```python
from build123d import *

# Parameters (mm, degrees)
F0_W     = 838.2
F0_H     = 457.2
F0_W_2   = 685.8
F0_H_2   = 304.8
F1_DEPTH = 22.225
F2_DEPTH = 9.525
F4_DEPTH = 6.35
F6_DEPTH = 6.35


with BuildPart() as f1:
    # F0 (on Front) → F1 (new body, symmetric)
    with BuildSketch(Plane.XZ):
        Rectangle(F0_W, F0_H)
        Rectangle(F0_W_2, F0_H_2, mode=Mode.SUBTRACT)
    extrude(amount=F1_DEPTH, both=True)

    # F0 (on Front) → F2 (join, symmetric)
    with BuildSketch(Plane.XZ):
        Rectangle(F0_W_2, F0_H_2)
    extrude(amount=F2_DEPTH, both=True)

    # F3 (on face) → F4 (join)
    with BuildSketch(Plane.XZ.offset(9.525)):
        Polygon((342.9, -152.4), (-189.5254737066, 152.4), (-342.9, 152.4), (189.5254737066, -152.4), align=None)
    extrude(amount=F4_DEPTH)

    # F5 (on face) → F6 (join)
    with BuildSketch(Plane.XZ.offset(9.525)):
        Polygon((-76.6872631467, 0), (-342.9, -152.4), (-189.5254737066, -152.4), (0, -43.90150164), align=None)
        Polygon((342.9, 152.4), (189.5254737066, 152.4), (0, 43.90150164), (76.6872631467, 0), align=None)
    extrude(amount=F6_DEPTH)


solid = f1.part
```
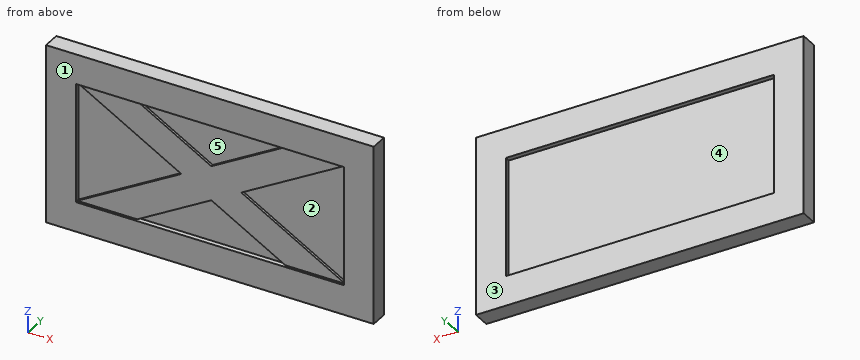
Could you check a few things on this model? Use its own coordinates, in mm. Face numbers are marked on the shaded views. A direction names the side the tool comes from. Round coordinates to 2 decimals unless told otherwise and drop trailing zeros. Loops run counter-clockwise (first coordinate to the right, second up) from the corner with the lowest first, then second, coordinate; pieces in that order, holes last. Notation, with made-up numbers: (62.5, 65) - (95.5, 65) arc R13 ccw to (95.5, 88) - close; hole circle Ø1 at (55, -35). An arc over 180 degrees is marked (long way). Answer in a Markdown table with one row per item. Add a question column.
(1) I need wall thicknesses on line 1 along Z through (x, y) = (-109, -20); line 2 along X through (y, z) = (20, -11.5); line 3 along X through (y, z) = (-10.5, 58.5). Which ranges of each line are inside material? Lowest first, please.
(2) If we section it at A-A (x = 40): Please give me the cut outline in (y, z) (3 decimals), plus the area to 3 significant figures.
(3) I'm going to push flat-ended pins straight in: pin 1 (6 mm diameter, centred on x = -141.5, z = 90, fed in from +Y) (3 decimals); pin 2 (2 mm diameter, centred on x = 33.5, z = 73.5, fed in from -Y) (3 decimals). Where does each tip first touch, or does it pass through?
(4) If we mould it in two halves opening along X, with no side actions, what happens to the marked faces 1 and 2? For each: pulls with the +X half, pulls with the -X half, needs draft (parallel to the pull), parting line crosses it, or undercut.
(5) For the marked faces 3, 4 and 5, which set-ups out of +Z, -Z, +X, -X, +Y, -Y let a thin tool reach every point of the face, with its end or its side?
(6) If we section it at B-B (z = 56.5): Please give me the cut outline in (x, y) (3 decimals), plus the area to 3 significant figures.
(7) If we section it at C-C (x = 158): Please give me the cut outline in (y, z) (3 decimals).
(8) If we section it at D-D (z = -28): Please give me the cut outline in (x, y) (3 decimals).
Model answer:
| question | item | result |
|---|---|---|
| 1 | line 1 | z = -228.6 to -152.4, 152.4 to 228.6 |
| 1 | line 2 | x = -419.1 to -342.9, 342.9 to 419.1 |
| 1 | line 3 | x = -419.1 to -342.9, -178.88 to -25.5, 25.5 to 178.88, 342.9 to 419.1 |
| 2 | outline | (-22.225, -228.6) - (22.225, -228.6) - (22.225, -152.4) - (9.525, -152.4) - (9.525, 152.4) - (22.225, 152.4) - (22.225, 228.6) - (-22.225, 228.6) - (-22.225, 152.4) - (-9.525, 152.4) - (-9.525, 66.8) - (-15.875, 66.8) - (-15.875, -66.8) - (-9.525, -66.8) - (-9.525, -152.4) - (-22.225, -152.4) - close |
| 2 | area | 13,400 mm² |
| 3 | pin 1 | stops at y = 9.525 |
| 3 | pin 2 | stops at y = -9.525 |
| 4 | face 1 | needs draft |
| 4 | face 2 | undercut |
| 5 | face 3 | +Z, -Z, +X, -X, +Y |
| 5 | face 4 | +Y |
| 5 | face 5 | -Y |
| 6 | outline | (-419.1, -22.225) - (-342.9, -22.225) - (-342.9, -9.525) - (-175.382, -9.525) - (-175.382, -15.875) - (-22.007, -15.875) - (-22.007, -9.525) - (22.007, -9.525) - (22.007, -15.875) - (175.382, -15.875) - (175.382, -9.525) - (342.9, -9.525) - (342.9, -22.225) - (419.1, -22.225) - (419.1, 22.225) - (342.9, 22.225) - (342.9, 9.525) - (-342.9, 9.525) - (-342.9, 22.225) - (-419.1, 22.225) - close |
| 6 | area | 21,800 mm² |
| 7 | outline | (-22.225, -228.6) - (22.225, -228.6) - (22.225, -152.4) - (9.525, -152.4) - (9.525, 152.4) - (22.225, 152.4) - (22.225, 228.6) - (-22.225, 228.6) - (-22.225, 152.4) - (-9.525, 152.4) - (-9.525, 134.352) - (-15.875, 134.352) - (-15.875, 46.549) - (-9.525, 46.549) - (-9.525, -46.549) - (-15.875, -46.549) - (-15.875, -134.352) - (-9.525, -134.352) - (-9.525, -152.4) - (-22.225, -152.4) - close |
| 8 | outline | (-419.1, -22.225) - (-342.9, -22.225) - (-342.9, -9.525) - (-125.598, -9.525) - (-125.598, -15.875) - (125.598, -15.875) - (125.598, -9.525) - (342.9, -9.525) - (342.9, -22.225) - (419.1, -22.225) - (419.1, 22.225) - (342.9, 22.225) - (342.9, 9.525) - (-342.9, 9.525) - (-342.9, 22.225) - (-419.1, 22.225) - close |
